from build123d import *

# Parameters (mm, degrees)
SKETCH_1_W          = 8
SKETCH_1_H          = 90
EXTRUDE_1_DEPTH     = 3
SKETCH_2_R          = 4
EXTRUDE_2_DEPTH     = 3
SKETCH_3_R          = 1.5
CUT_EXTRUDE_1_DEPTH = 3


with BuildPart() as part:
    # 草图1 → 凸台-拉伸1 (new body)
    with BuildSketch(Plane.XY):
        Rectangle(SKETCH_1_W, SKETCH_1_H)
    extrude(amount=EXTRUDE_1_DEPTH)

    # 草图2 → 凸台-拉伸2 (add)
    with BuildSketch(Plane.XY):
        with Locations((0, 45)):
            Circle(SKETCH_2_R)
        with Locations((0, -45)):
            Circle(SKETCH_2_R)
    extrude(amount=EXTRUDE_2_DEPTH)

    # 草图3 → 切除-拉伸1 (cut)
    with BuildSketch(Plane.XY.offset(3)):
        with Locations((0, 45)):
            Circle(SKETCH_3_R)
        with Locations((0, -45)):
            Circle(SKETCH_3_R)
    extrude(amount=-CUT_EXTRUDE_1_DEPTH, mode=Mode.SUBTRACT)


solid = part.part
Can you work these out from the model? Positions are in its coordinate system, mm. Coordinates: 2 decimals unless noted, no trailing zeros. Loops run counter-clockwise (first coordinate to the right, second up) from the corner with the lowest first, then second, coordinate; pieces in that order, holes last. Notation, with made-up numbers: (61, -30) - (119, -30) arc R20 ccw to (119, -19) - close; hole circle Ø9 at (-14, -9). An arc over 180 degrees is marked (long way). Answer as a JSON object with one key per item and string values. Group by question number.
Item 1: If we mould it in two halves opening along X, with no side actions, what happens to faces 1 (the face through (0, 49, 1)), 2 (the face through (0, 1, 0)), 3 (the face through (-0.325, 43.536, 1.521))? For each: released by +X, released by -X, zero draft, split by the parting line, or undercut.
Item 2: If I drill on L1, parallel to Y at x = 0, z = 0.7; L2, parallel to Y at x = 1, z = 0.3; L3, parallel to Y at x = 1.75, z = 1.2, over which ranges is the centre line in solid material (lowest first)? Write a range as from..to.
Item 3: If we section it at B-B (z = 0.95): List the corners of the cut face in (x, y) for me.
Item 4: If we section it at A-A (x = 0): List the corners of the cut face in (y, z) for me.
Returned:
{
 "1": {"face 1": "split by the parting line", "face 2": "zero draft", "face 3": "undercut"},
 "2": {"L1": "y = -49..-46.5, -43.5..43.5, 46.5..49", "L2": "y = -48.87..-46.12, -43.88..43.88, 46.12..48.87", "L3": "y = -48.6..48.6"},
 "3": {"outline": "(-4, -45) arc R4 ccw to (4, -45) - (4, 45) arc R4 ccw to (-4, 45) - close; hole circle Ø3 at (0, -45); hole circle Ø3 at (0, 45)"},
 "4": {"outline": "(-49, 0) - (-46.5, 0) - (-46.5, 3) - (-49, 3) - close; (-43.5, 0) - (43.5, 0) - (43.5, 3) - (-43.5, 3) - close; (46.5, 0) - (49, 0) - (49, 3) - (46.5, 3) - close"}
}
